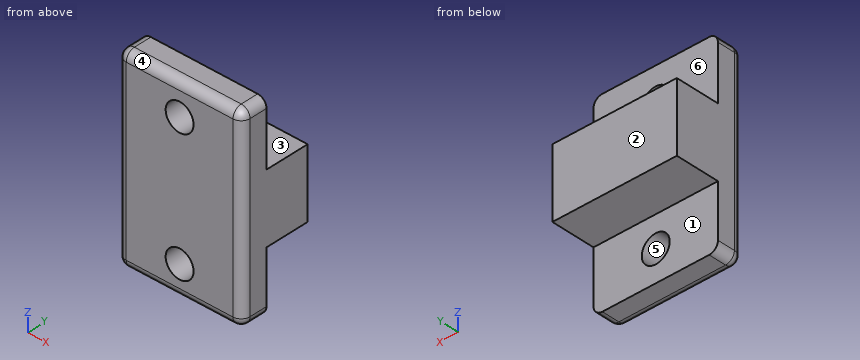
```python
from build123d import *

# Parameters (mm, degrees)
SKETCH_1_W          = 14.05
SKETCH_1_H          = 7.85
EXTRUDE_1_DEPTH     = 5
EXTRUDE_2_DEPTH     = 3
SKETCH_3_R          = 1.575
CUT_EXTRUDE_1_DEPTH = 3
FILLET_2_R          = 1


with BuildPart() as part:
    # 草图1 → 凸台-拉伸1 (new body)
    with BuildSketch(Plane(origin=(0, 0, 0), x_dir=(1, 0, 0), z_dir=(0, 1, 0))):
        Rectangle(SKETCH_1_W, SKETCH_1_H)
    extrude(amount=EXTRUDE_1_DEPTH)

    # 草图2 → 凸台-拉伸2 (add)
    with BuildSketch(Plane(origin=(0, 0, 0), x_dir=(-1, 0, 0), z_dir=(0, -1, 0))):
        Polygon((-7.025, 3.925), (-7.025, 10.9), (7.025, 10.9), (7.025, 3.925), (7.025, -11.1), (-7.025, -11.1), align=None)
    extrude(amount=EXTRUDE_2_DEPTH)

    # 草图3 → 切除-拉伸1 (cut)
    with BuildSketch(Plane(origin=(0, 0, 0), x_dir=(1, 0, 0), z_dir=(0, 1, 0))):
        with Locations(Location((0, 7.4125, 0), (0, 0, 270))):
            Circle(SKETCH_3_R)
    cut_extrude_1 = extrude(amount=-CUT_EXTRUDE_1_DEPTH, mode=Mode.SUBTRACT)

    # 镜向1: 切除-拉伸1 across plane
    add(cut_extrude_1.mirror(Plane.XY), mode=Mode.SUBTRACT)

    # 圆角2
    fillet_2_edges = [part.edges().sort_by_distance(p)[0] for p in [
        (7.025, -1.5, 11.1),
        (-7.025, -1.5, 11.1),
        (-7.025, -1.5, -10.9),
        (7.025, -1.5, -10.9),
        (7.025, -3, 0.1),
        (0, -3, 11.1),
        (-7.025, -3, 0.1),
        (0, -3, -10.9),
    ]]
    fillet(fillet_2_edges, radius=FILLET_2_R)


solid = part.part
```
Here's how the part is built. I have some questions about the finished solid (model axes, mm). Face numbers are marked on the shaded views. A direction names the side the tool comes from. Round coordinates to 2 decimals unless told otherwise and drop trailing zeros. Order: outer loops, then holes, each group sorted by start corner. A loop starts at its lowest first (then second) coordinate and runs counter-clockwise, first axis right, second up. Notation, with made-up numbers: (53, 82.25) -> (86, 82.25) arc R19 ccw to (86, 99.25) -> close; hole circle Ø11 at (-35.5, 87). An arc over 180 degrees is marked (long way). Use a Markdown table: item, result. Add a question column.
(1) For the marked faces 1, 2 and 3, which set-ups out of +Z, -Z, +X, -X, +Y, -Y let a thin tool reach every point of the face, with its end or its side?
(2) Suppose I cut it at D-D, the plane y = 3.75. Please give me the cut outline in (x, z) (3 decimals), and give its area (3 significant figures).
(3) Suppose I cut it at B-B, the plane z = -8. Please give me the cut outline in (x, y) (3 decimals).
(4) Suppose I cut it at A-A, the plane x = 0. Please give me the cut outline in (y, z) (1 decimal), and give its area (3 significant figures).
(5) I need wall thicknesses on line 1 along Y through (x, z) = (-3, 9.75); line 2 along Z through (x, y) = (-1.25, 1.75) (3 decimals); line 3 along X through (y, z) = (-1.5, 6.25) (3 decimals). Which ranges of each line are inside material? Lowest first, please.
(6) For pin 1 Ø4 at (x, z) = (0, 7.41) entering from +Y, with a flat end and sliding along its axis, tell me the tip position at first contact or that it passes through.
(7) Suppose I cut it at C-C, the plane x = 4.25. Please give me the cut outline in (y, z) (3 decimals), and give its area (3 significant figures).
(8) If we mould it in two halves opening along Z, with no side actions, what happens to the marked faces 4, 5 and 6? For each: released by +Z, released by -Z, zero draft, split by the parting line, or undercut.
Verdict:
| question | item | result |
|---|---|---|
| 1 | face 1 | -Z, +X, -X, +Y |
| 1 | face 2 | +Z, -Z, +X, -X, +Y |
| 1 | face 3 | +Z, +X, -X, +Y |
| 2 | outline | (-7.025, -3.925) -> (7.025, -3.925) -> (7.025, 3.925) -> (-7.025, 3.925) -> close |
| 2 | area | 110 mm2 |
| 3 | outline | (-7.025, -2) arc R1 ccw to (-6.025, -3) -> (-1.461, -3) -> (-1.461, 0) -> (-7.025, 0) -> close; (1.461, -3) -> (6.025, -3) arc R1 ccw to (7.025, -2) -> (7.025, 0) -> (1.461, 0) -> close |
| 4 | outline | (-3, -9.9) arc R1 ccw to (-2, -10.9) -> (0, -10.9) -> (0, -9) -> (-3, -9) -> close; (-3, -5.8) -> (0, -5.8) -> (0, -3.9) -> (5, -3.9) -> (5, 3.9) -> (0, 3.9) -> (0, 5.8) -> (-3, 5.8) -> close; (-3, 9) -> (0, 9) -> (0, 11.1) -> (-2, 11.1) arc R1 ccw to (-3, 10.1) -> close |
| 4 | area | 85.9 mm2 |
| 5 | line 1 | -3 to 0 |
| 5 | line 2 | -3.925 to 3.925 |
| 5 | line 3 | -7.025 to -1.063, 1.063 to 7.025 |
| 6 | pin 1 | y = 0 |
| 7 | outline | (-3, -9.9) arc R1 ccw to (-2, -10.9) -> (0, -10.9) -> (0, -3.925) -> (5, -3.925) -> (5, 3.925) -> (0, 3.925) -> (0, 11.1) -> (-2, 11.1) arc R1 ccw to (-3, 10.1) -> close |
| 7 | area | 105 mm2 |
| 8 | face 4 | released by +Z |
| 8 | face 5 | undercut |
| 8 | face 6 | zero draft |
